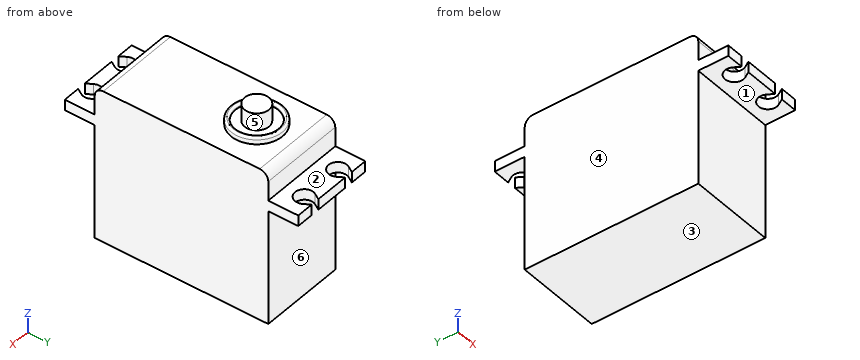
from build123d import *

# Parameters (mm, degrees)
BOSS_EXTRUDE1_DEPTH = 10
SKETCH3_R           = 2.15
CUT_EXTRUDE2_DEPTH  = 2.5
SKETCH2_R           = 6
BOSS_EXTRUDE2_DEPTH = 1.55
CUT_EXTRUDE1_START  = 1.55
CUT_EXTRUDE1_DEPTH  = 0.8
SKETCH2_4_R         = 2.86
BOSS_EXTRUDE3_DEPTH = 4.77
FILLET1_R           = 0.5


with BuildPart() as part:
    # Sketch1 → Boss-Extrude1 (new, symmetric)
    with BuildSketch(Plane(origin=(0, 0, 0), x_dir=(0, 0, -1), z_dir=(1, 0, 0))):
        with BuildLine():
            Line((35.88, -20.25), (35.88, 20.25))
            Line((35.88, 20.25), (9.03, 20.25))
            Line((9.03, 20.25), (9.03, 27.25))
            Line((9.03, 27.25), (6.53, 27.25))
            Line((6.53, 27.25), (6.53, 20.25))
            Line((6.53, 20.25), (2, 20.25))
            ThreePointArc((2, 20.25), (0.585786438, 19.664213562), (0, 18.25))
            Line((0, 18.25), (0, -18.25))
            ThreePointArc((0, -18.25), (0.585786438, -19.664213562), (2, -20.25))
            Line((2, -20.25), (6.53, -20.25))
            Line((6.53, -20.25), (6.53, -27.25))
            Line((6.53, -27.25), (9.03, -27.25))
            Line((9.03, -27.25), (9.03, -20.25))
            Line((9.03, -20.25), (35.88, -20.25))
        make_face()
    extrude(amount=BOSS_EXTRUDE1_DEPTH, both=True)

    # Sketch3 → Cut-Extrude2 (cut)
    with BuildSketch(Plane.XY.offset(-6.53)):
        with Locations((-5, 24.75)):
            Circle(SKETCH3_R)
        with BuildLine():
            Line((-6, 27.25), (-6.839329825, 25.86326807))
            ThreePointArc((-6.839329825, 25.86326807), (-5, 26.9), (-3.160670175, 25.86326807))
            Line((-3.160670175, 25.86326807), (-4, 27.25))
            Line((-4, 27.25), (-6, 27.25))
        make_face()
        with Locations((5, 24.75)):
            Circle(SKETCH3_R)
        with BuildLine():
            Line((6, 27.25), (4, 27.25))
            Line((4, 27.25), (3.160670175, 25.86326807))
            ThreePointArc((3.160670175, 25.86326807), (5, 26.9), (6.839329825, 25.86326807))
            Line((6.839329825, 25.86326807), (6, 27.25))
        make_face()
    cut_extrude2 = extrude(amount=-CUT_EXTRUDE2_DEPTH, mode=Mode.SUBTRACT)

    # Sketch2 → Boss-Extrude2 (add)
    with BuildSketch(Plane.XY):
        with Locations(Location((0, 9.75, 0), (0, 0, 90))):
            Circle(SKETCH2_R)
    extrude(amount=BOSS_EXTRUDE2_DEPTH)

    # Sketch2<3> → Cut-Extrude1 (cut)
    with BuildSketch(Plane.XY.offset(CUT_EXTRUDE1_START)):
        with BuildLine():
            ThreePointArc((-2.86, 9.75), (0, 12.61), (2.86, 9.75))
            Line((2.86, 9.75), (5, 9.75))
            ThreePointArc((5, 9.75), (0, 14.75), (-5, 9.75))
            Line((-5, 9.75), (-2.86, 9.75))
        make_face()
        with BuildLine():
            Line((5, 9.75), (2.86, 9.75))
            ThreePointArc((2.86, 9.75), (0, 6.89), (-2.86, 9.75))
            Line((-2.86, 9.75), (-5, 9.75))
            ThreePointArc((-5, 9.75), (0, 4.75), (5, 9.75))
        make_face()
        with BuildLine():
            ThreePointArc((-2.86, 9.75), (0, 6.89), (2.86, 9.75))
            Line((2.86, 9.75), (-2.86, 9.75))
        make_face()
        with BuildLine():
            Line((-2.86, 9.75), (2.86, 9.75))
            ThreePointArc((2.86, 9.75), (0, 12.61), (-2.86, 9.75))
        make_face()
    extrude(amount=-CUT_EXTRUDE1_DEPTH, mode=Mode.SUBTRACT)

    # Sketch2<4> → Boss-Extrude3 (add)
    with BuildSketch(Plane.XY):
        with Locations((0, 9.75)):
            Circle(SKETCH2_4_R)
    extrude(amount=BOSS_EXTRUDE3_DEPTH)

    # Mirror1: Cut-Extrude2 across plane
    add(cut_extrude2.mirror(Plane.ZX), mode=Mode.SUBTRACT)

    # Fillet1
    fillet1_edges = [part.edges().sort_by_distance(p)[0] for p in [
        (0, 3.75, 1.55),
        (5, 9.75, 1.55),
    ]]
    fillet(fillet1_edges, radius=FILLET1_R - 0.0001)  # a hair under: the kernel refuses the full size


solid = part.part
Source: CAD feature listing. Evaluate the final solid. Frame: model axes, mm. Face numbers are marked on the shaded views. A direction names the side the tool comes from. Coordinates: 2 decimals unless noted, no trailing zeros. Loops run counter-clockwise (first coordinate to the right, second up) from the corner with the lowest first, then second, coordinate; pieces in that order, holes last. Notation, with made-up numbers: (85, 58) - (96, 58) arc R33 cw to (96, 86) - close; hole circle Ø2 at (-22, 54.5). An arc over 180 degrees is marked (long way). One line per item, written item: value. Start each with the question number.
1. Ray query, L1, parallel to X at y = 24.75, z = -7.45; L2, parallel to Y at x = -5.5, z = -20.5; L3, parallel to Z at x = 5.5, y = 3. Return the intervals inside material, ascending.
2. Section D-D (y = -21). Return the cut outline in (x, z).
3. Mould query, pull axis X, two halves, no side actions, for the marked faces 4, 5 and 6. Classes: pulls with the +X half, pulls with the -X half, needs draft (parallel to the pull), parting line crosses it, or undercut.
4. Section C-C (z = -22). Return the cut outline in (x, y).
5. Section A-A (y = 24.75). Return the cut outline in (x, z).
6. Contact query for flat-ended pins moving along their axis: P1, Ø6, axis at x = 2, y = 5, coming from the +Z side; P2, Ø2.5, axis at x = -2, z = -5, coming from the -Y side; P3, Ø10, axis at x = 3.5, z = -23.5, coming from the +Y side; P4, Ø5.5, axis at x = 5, y = -24.75, coming from the -Z side. Output: stop coordinate, or through.
7. Set-up query: the marked faces 1, 2 and 3. Return all of +Z, -Z, +X, -X, +Y, -Y with unobstructed straight access to the full face (end or side cutting, diameter ignored); none if empty.
Verdict:
1. L1: x = -10 to -7.15, -2.85 to 2.85, 7.15 to 10
1. L2: y = -20.25 to 20.25
1. L3: z = -35.88 to 0
2. outline: (-10, -9.03) - (10, -9.03) - (10, -6.53) - (-10, -6.53) - close
3. face 4: pulls with the -X half
3. face 5: undercut
3. face 6: needs draft
4. outline: (-10, -20.25) - (10, -20.25) - (10, 20.25) - (-10, 20.25) - close
5. outline: (-10, -9.03) - (-7.15, -9.03) - (-7.15, -6.53) - (-10, -6.53) - close; (-2.85, -9.03) - (2.85, -9.03) - (2.85, -6.53) - (-2.85, -6.53) - close; (7.15, -9.03) - (10, -9.03) - (10, -6.53) - (7.15, -6.53) - close
6. P1: stops at z = 4.77
6. P2: stops at y = -20.25
6. P3: stops at y = 20.25
6. P4: stops at z = -9.03
7. face 1: -Z, +X, -X, -Y
7. face 2: +Z, +X, -X, +Y
7. face 3: -Z, +X, -X, +Y, -Y
